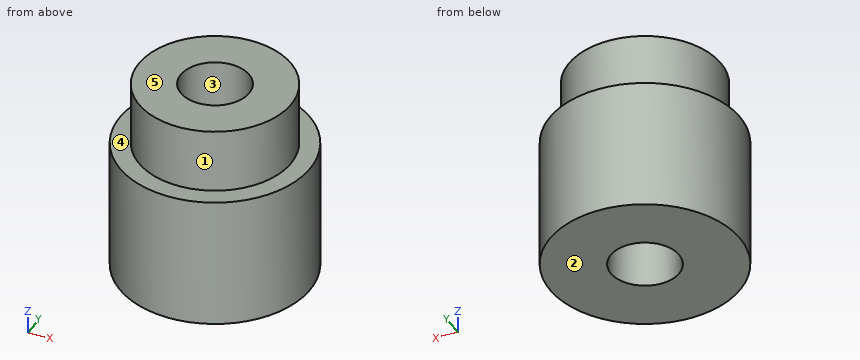
from build123d import *

# Parameters (mm, degrees)
CYLINDER002_R     = 0.9
CYLINDER002_DEPTH = 10
CYLINDER_R        = 2.5
CYLINDER_DEPTH    = 3.5
CYLINDER001_R     = 2
CYLINDER001_DEPTH = 5.2


with BuildPart() as cylinder002:
    # Cylinder002 → Cylinder002 (new body)
    with BuildSketch(Plane.XY):
        Circle(CYLINDER002_R)
    extrude(amount=CYLINDER002_DEPTH)


with BuildPart() as cylinder:
    # Cylinder → Cylinder (new body)
    with BuildSketch(Plane.XY):
        Circle(CYLINDER_R)
    extrude(amount=CYLINDER_DEPTH)


with BuildPart() as obj1:
    # Cylinder001 → Cylinder001 (new body)
    with BuildSketch(Plane.XY):
        Circle(CYLINDER001_R)
    extrude(amount=CYLINDER001_DEPTH)

    # Fusion: union Cylinder
    add(cylinder.part)

    # Cut: cut Cylinder002
    add(cylinder002.part, mode=Mode.SUBTRACT)


solid = obj1.part
Check sheet for the modelled part. Datum: model origin and axes. Units: mm. Face numbers are marked on the shaded views. A direction names the side the tool comes from. Give positions to 0.01 mm unless a question says otherwise; leave off trailing zeros. Loops run counter-clockwise (first coordinate to the right, second up) from the corner with the lowest first, then second, coordinate; pieces in that order, holes last. Notation, with made-up numbers: M 14.25,52 L 60.25,52 A25 ccw 60.25,81 Z; hole C -34.5,-31 d4. An arc over 180 degrees is marked long. Use a Markdown table: item, result. Add a question column.
Q1. Sectioned sample at A-A, the plane y = 0. Record the cut outline in (x, z).
Q2. Mould release check, pull along Y, two halves, no side actions. Record for the marked faces 1, 2 and 3: pulls with the +Y half, pulls with the -Y half, needs draft (parallel to the pull), parting line crosses it, or undercut.
Q3. Sectioned sample at C-C, the plane z = 4.45. Record the cut outline in (x, y), then the cut area to 3 significant figures.
Q4. Go/stop test with flat-tipped pins: pin 1 (1.5 mm diameter, centred on x = -1.5, z = 2.5, fed in from +Y); pin 2 (3 mm diameter, centred on x = 2, z = 3.5, fed in from -Y). Record where each tip stops, or that it passes through.
Q5. Tool access check on the marked faces 4 and 5. Record the directions out of +Z, -Z, +X, -X, +Y, -Y that give a thin tool (end or side, any length) a straight path to the whole face; none if there is none.
Q6. Scan lines: line 1 along Y through (x, z) = (0, 4.15); line 2 along Y through (x, z) = (0, 3.2); line 3 along Z through (x, y) = (-1.55, -1.75). Record each from-to range of solid material in increasing order. Write a range as [from, to].
Q7. Sectioned sample at D-D, the plane x = 1.3. Record the cut outline in (y, z).
Verdict:
| question | item | result |
|---|---|---|
| 1 | outline | M -2.5,0 L -0.9,0 L -0.9,5.2 L -2,5.2 L -2,3.5 L -2.5,3.5 Z; M 0.9,0 L 2.5,0 L 2.5,3.5 L 2,3.5 L 2,5.2 L 0.9,5.2 Z |
| 2 | face 1 | parting line crosses it |
| 2 | face 2 | needs draft |
| 2 | face 3 | undercut |
| 3 | outline | C 0,0 d4; hole C 0,0 d1.8 |
| 3 | area | 10.0 mm^2 |
| 4 | pin 1 | y = 2.38 |
| 4 | pin 2 | y = -2.45 |
| 5 | face 4 | +Z |
| 5 | face 5 | +Z, +X, -X, +Y, -Y |
| 6 | line 1 | [-2, -0.9], [0.9, 2] |
| 6 | line 2 | [-2.5, -0.9], [0.9, 2.5] |
| 6 | line 3 | [0, 3.5] |
| 7 | outline | M -2.14,0 L 2.14,0 L 2.14,3.5 L 1.52,3.5 L 1.52,5.2 L -1.52,5.2 L -1.52,3.5 L -2.14,3.5 Z |
